Check sheet for the drawn part. Datum: minimum x, y, z corner. Units: mm. Give positions to 0.01 mm unless a question says otherwise; leave off trailing zeros. Loops run counter-clockwise (first coordinate to the right, second up) from the corner with the lowest first, then second, coordinate; pieces in that order, holes last.
1. Cross-section at A-A, the plane y = 18. Record the cut outline in (x, z), plus the area to 3 significant figures.
2. Cross-section at B-B, the plane z = 32. Record the cut outline in (x, y), plus the area to 3 significant figures.
3. Go/stop test with flat-tipped pins: pin 1 Ø2.5 at (x, z) = (12.5, 8) entering from +Y; pin 2 Ø4 at (x, z) = (12.5, 18) entering from +Y; pin 3 Ø3.5 at (x, z) = (12.5, 22) entering from +Y; pin 4 Ø3 at (x, z) = (4, 25) entering from +Y. Record where each tip stops, or that it passes through.
4. Material ranges on L1, parallel to Z at x = 12.5, y = 16.25; L2, parallel to Z at x = 13.5, y = 21; L3, parallel to X at y = 4.25, z = 31, recorded low to high.
5. Cross-section at C-C, the plane x = 5. Record the cut outline in (y, z), plus the area to 3 significant figures.
6. Cross-section at D-D, the plane z = 5. Record the cut outline in (x, y).
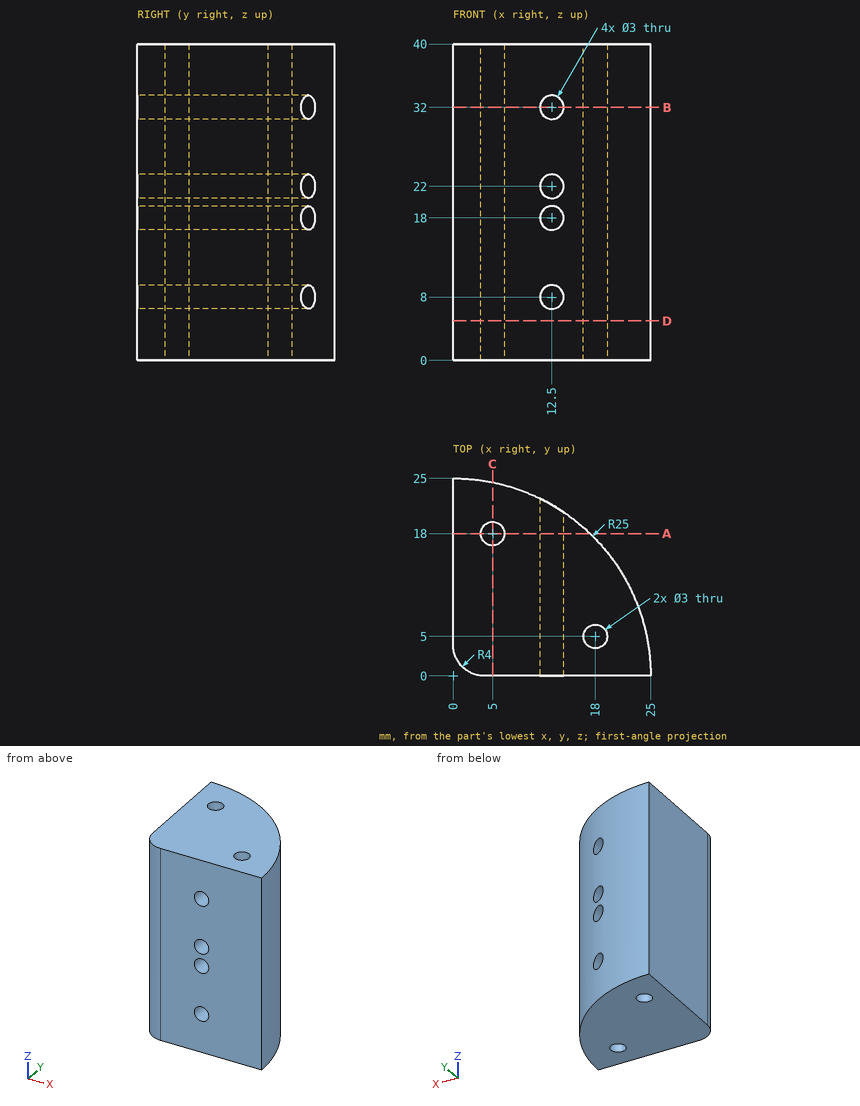
Result:
1. outline: (0, 0) - (3.5, 0) - (3.5, 40) - (0, 40) - close; (6.5, 0) - (17.35, 0) - (17.35, 40) - (6.5, 40) - close; hole circle Ø3 at (12.5, 8); hole circle Ø3 at (12.5, 18); hole circle Ø3 at (12.5, 22); hole circle Ø3 at (12.5, 32)
1. area: 546 mm2
2. outline: (0, 4) arc R4 ccw to (4, 0) - (11, 0) - (11, 22.45) arc R25 ccw to (0, 25) - close; (14, 0) - (25, 0) arc R25 ccw to (14, 20.71) - close; hole circle Ø3 at (5, 18); hole circle Ø3 at (18, 5)
2. area: 408 mm2
3. pin 1: passes through
3. pin 2: stops at y = 22.69
3. pin 3: stops at y = 22.57
3. pin 4: stops at y = 24.87
4. L1: z = 0 to 6.5, 9.5 to 16.5, 19.5 to 20.5, 23.5 to 30.5, 33.5 to 40
4. L2: z = 0 to 6.88, 9.12 to 16.88, 19.12 to 20.88, 23.12 to 30.88, 33.12 to 40
4. L3: x = 0 to 11.38, 13.62 to 16.7, 19.3 to 24.64
5. outline: (0, 0) - (16.5, 0) - (16.5, 40) - (0, 40) - close; (19.5, 0) - (24.49, 0) - (24.49, 40) - (19.5, 40) - close
5. area: 860 mm2
6. outline: (0, 4) arc R4 ccw to (4, 0) - (25, 0) arc R25 ccw to (0, 25) - close; hole circle Ø3 at (5, 18); hole circle Ø3 at (18, 5)
